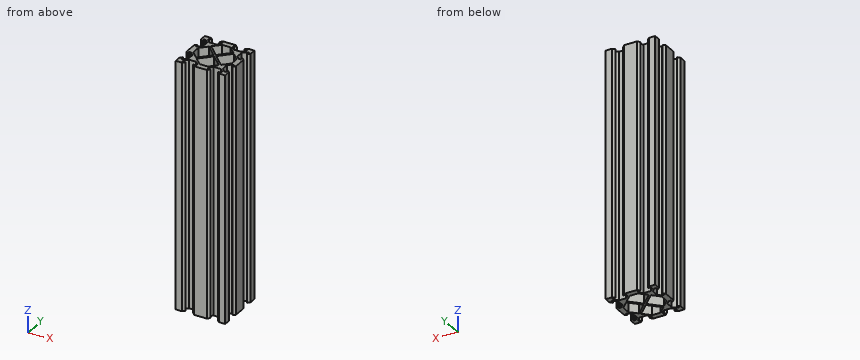
```python
from build123d import *

# Parameters (mm, degrees)
SKETCH2_W              = 20
SKETCH2_H              = 20
BOSS_EXTRUDE1_DEPTH    = 200
CUT_EXTRUDE1_DEPTH     = 201.499376558
CIRPATTERN2_COUNT      = 4
LPATTERN1_COUNT        = 2
LPATTERN1_PITCH        = 20
LPATTERN1_COUNT_DIR2   = 2
LPATTERN1_PITCH_DIR2   = 20
LPATTERN1_COPY_1_DEPTH = 201.499376558
LPATTERN1_COPY_2_DEPTH = 201.499376558
LPATTERN1_COPY_3_DEPTH = 201.499376558
LPATTERN1_COPY_4_DEPTH = 201.499376558
LPATTERN1_COPY_5_DEPTH = 201.499376558
LPATTERN1_COPY_6_DEPTH = 201.499376558
LPATTERN1_COPY_7_DEPTH = 201.499376558
LPATTERN1_COPY_8_DEPTH = 201.499376558
LPATTERN1_COPY_9_DEPTH = 201.499376558
CUT_EXTRUDE2_DEPTH     = 205.450483003


with BuildPart() as part:
    # Sketch2 → Boss-Extrude1 (new body)
    with BuildSketch(Plane.XY):
        Rectangle(SKETCH2_W, SKETCH2_H)
    boss_extrude1 = extrude(amount=-BOSS_EXTRUDE1_DEPTH)

    # Sketch3 → Cut-Extrude1 (cut, symmetric)
    with BuildSketch(Plane.XY):
        Polygon((-3.1, 8.2), (-4.9, 10), (4.9, 10), (3.1, 8.2), (5.5, 8.2), (5.5, 6.56), (2.84, 3.9), (-2.84, 3.9), (-5.5, 6.56), (-5.5, 8.2), align=None)
    cut_extrude1 = extrude(amount=CUT_EXTRUDE1_DEPTH, both=True, mode=Mode.SUBTRACT)

    # CirPattern2: Cut-Extrude1 ×4 about axis
    cirpattern2_axis = Axis((0, 0, 0), (0, 0, 1))
    for i in range(1, CIRPATTERN2_COUNT):
        add(cut_extrude1.rotate(cirpattern2_axis, i * 360 / CIRPATTERN2_COUNT), mode=Mode.SUBTRACT)

    # LPattern1: Boss-Extrude1, Cut-Extrude1 2 × 2
    with Locations(*[(j * LPATTERN1_PITCH_DIR2, i * LPATTERN1_PITCH, 0) for i in range(LPATTERN1_COUNT) for j in range(LPATTERN1_COUNT_DIR2) if (i, j) != (0, 0)]):
        add(boss_extrude1)
        add(cut_extrude1, mode=Mode.SUBTRACT)

    # LPattern1 copy 1 sketch → LPattern1 copy 1 (cut, symmetric)
    with BuildSketch(Plane(origin=(20, 0, 0), x_dir=(0, 1, 0), z_dir=(0, 0, 1))):
        Polygon((-3.1, 8.2), (-4.9, 10), (4.9, 10), (3.1, 8.2), (5.5, 8.2), (5.5, 6.56), (2.84, 3.9), (-2.84, 3.9), (-5.5, 6.56), (-5.5, 8.2), align=None)
    extrude(amount=LPATTERN1_COPY_1_DEPTH, both=True, mode=Mode.SUBTRACT)

    # LPattern1 copy 2 sketch → LPattern1 copy 2 (cut, symmetric)
    with BuildSketch(Plane(origin=(0, 20, 0), x_dir=(0, 1, 0), z_dir=(0, 0, 1))):
        Polygon((-3.1, 8.2), (-4.9, 10), (4.9, 10), (3.1, 8.2), (5.5, 8.2), (5.5, 6.56), (2.84, 3.9), (-2.84, 3.9), (-5.5, 6.56), (-5.5, 8.2), align=None)
    extrude(amount=LPATTERN1_COPY_2_DEPTH, both=True, mode=Mode.SUBTRACT)

    # LPattern1 copy 3 sketch → LPattern1 copy 3 (cut, symmetric)
    with BuildSketch(Plane(origin=(20, 20, 0), x_dir=(0, 1, 0), z_dir=(0, 0, 1))):
        Polygon((-3.1, 8.2), (-4.9, 10), (4.9, 10), (3.1, 8.2), (5.5, 8.2), (5.5, 6.56), (2.84, 3.9), (-2.84, 3.9), (-5.5, 6.56), (-5.5, 8.2), align=None)
    extrude(amount=LPATTERN1_COPY_3_DEPTH, both=True, mode=Mode.SUBTRACT)

    # LPattern1 copy 4 sketch → LPattern1 copy 4 (cut, symmetric)
    with BuildSketch(Plane(origin=(20, 0, 0), x_dir=(-1, 0, 0), z_dir=(0, 0, 1))):
        Polygon((-3.1, 8.2), (-4.9, 10), (4.9, 10), (3.1, 8.2), (5.5, 8.2), (5.5, 6.56), (2.84, 3.9), (-2.84, 3.9), (-5.5, 6.56), (-5.5, 8.2), align=None)
    extrude(amount=LPATTERN1_COPY_4_DEPTH, both=True, mode=Mode.SUBTRACT)

    # LPattern1 copy 5 sketch → LPattern1 copy 5 (cut, symmetric)
    with BuildSketch(Plane(origin=(0, 20, 0), x_dir=(-1, 0, 0), z_dir=(0, 0, 1))):
        Polygon((-3.1, 8.2), (-4.9, 10), (4.9, 10), (3.1, 8.2), (5.5, 8.2), (5.5, 6.56), (2.84, 3.9), (-2.84, 3.9), (-5.5, 6.56), (-5.5, 8.2), align=None)
    extrude(amount=LPATTERN1_COPY_5_DEPTH, both=True, mode=Mode.SUBTRACT)

    # LPattern1 copy 6 sketch → LPattern1 copy 6 (cut, symmetric)
    with BuildSketch(Plane(origin=(20, 20, 0), x_dir=(-1, 0, 0), z_dir=(0, 0, 1))):
        Polygon((-3.1, 8.2), (-4.9, 10), (4.9, 10), (3.1, 8.2), (5.5, 8.2), (5.5, 6.56), (2.84, 3.9), (-2.84, 3.9), (-5.5, 6.56), (-5.5, 8.2), align=None)
    extrude(amount=LPATTERN1_COPY_6_DEPTH, both=True, mode=Mode.SUBTRACT)

    # LPattern1 copy 7 sketch → LPattern1 copy 7 (cut, symmetric)
    with BuildSketch(Plane(origin=(20, 0, 0), x_dir=(0, -1, 0), z_dir=(0, 0, 1))):
        Polygon((-3.1, 8.2), (-4.9, 10), (4.9, 10), (3.1, 8.2), (5.5, 8.2), (5.5, 6.56), (2.84, 3.9), (-2.84, 3.9), (-5.5, 6.56), (-5.5, 8.2), align=None)
    extrude(amount=LPATTERN1_COPY_7_DEPTH, both=True, mode=Mode.SUBTRACT)

    # LPattern1 copy 8 sketch → LPattern1 copy 8 (cut, symmetric)
    with BuildSketch(Plane(origin=(0, 20, 0), x_dir=(0, -1, 0), z_dir=(0, 0, 1))):
        Polygon((-3.1, 8.2), (-4.9, 10), (4.9, 10), (3.1, 8.2), (5.5, 8.2), (5.5, 6.56), (2.84, 3.9), (-2.84, 3.9), (-5.5, 6.56), (-5.5, 8.2), align=None)
    extrude(amount=LPATTERN1_COPY_8_DEPTH, both=True, mode=Mode.SUBTRACT)

    # LPattern1 copy 9 sketch → LPattern1 copy 9 (cut, symmetric)
    with BuildSketch(Plane(origin=(20, 20, 0), x_dir=(0, -1, 0), z_dir=(0, 0, 1))):
        Polygon((-3.1, 8.2), (-4.9, 10), (4.9, 10), (3.1, 8.2), (5.5, 8.2), (5.5, 6.56), (2.84, 3.9), (-2.84, 3.9), (-5.5, 6.56), (-5.5, 8.2), align=None)
    extrude(amount=LPATTERN1_COPY_9_DEPTH, both=True, mode=Mode.SUBTRACT)

    # Sketch9 → Cut-Extrude2 (cut, through all)
    with BuildSketch(Plane.XY):
        Polygon((1.06, 0), (6.56, -5.5), (13.44, -5.5), (18.94, 0), (10, 8.94), align=None)
        Polygon((20, 1.06), (25.5, 6.56), (25.5, 11.8), (25.5, 13.44), (20, 18.94), (11.06, 10), align=None)
        Polygon((0, 1.06), (8.94, 10), (0, 18.94), (-5.5, 13.44), (-5.5, 6.56), align=None)
        Polygon((1.06, 20), (10, 11.06), (18.94, 20), (13.44, 25.5), (6.56, 25.5), align=None)
    extrude(amount=-CUT_EXTRUDE2_DEPTH, mode=Mode.SUBTRACT)


solid = part.part
```
The listing builds one solid part. Answer for the finished solid, in the listing's coordinates (mm). Round coordinates to 2 decimals unless told otherwise and drop trailing zeros. Put each result on its own line as item: value. Start each with the question number.
(1) Straight lines are drawn through the part: probe 1 along X at (y, z) = (-6, -151); probe 2 along Y at (x, z) = (22, -9.5); probe 3 along Y at (x, z) = (2.5, -98). For each, find the intervals that lie inside material, in ascending order. Write a range as from..to.
(2) Find section A-A (z = -134.5). State how many separate pieces and enclosed holes the cut face has, plus the area to 3 significant figures.
(3) Given P1, Ø6, axis at y = -1.5, z = -74, coming from the +X side; P2, Ø6, axis at y = 21, z = -103, coming from the +X side; P3, Ø1.5, axis at x = 16.5, z = -99, coming from the -Y side, each flat-ended and moving along its own axis, determine where each tip first touches the part or whether it passes through.
Reply:
1. probe 1: -10..-4.94, 4.94..15.06, 24.94..30
1. probe 2: -3.9..3.06, 16.94..23.9
1. probe 3: -3.9..-1.44, 1.44..3.56, 16.44..18.56, 21.44..23.9
2. separate pieces: 1
2. enclosed holes: 4
2. area: 571 mm^2
3. P1: x = 29.6
3. P2: x = 29.1
3. P3: y = -9.35
